Geometry: final body of the model. Coordinates: model frame, mm. A direction names the side the tool comes from. Round coordinates to 2 decimals unless told otherwise and drop trailing zeros. Loops run counter-clockwise (first coordinate to the right, second up) from the corner with the lowest first, then second, coordinate; pieces in that order, holes last. Notation, with made-up numbers: M -17,13.5 L 18,13.5 A18 cw 18,28.5 Z; hole C -34.75,-36.5 d10. An arc over 180 degrees is marked long. Return JSON: item names as keys, results as strings.
from build123d import *

# Parameters (mm, degrees)
F0_R     = 12.4944504689
F1_DEPTH = 25
F3_DEPTH = 20
F4_R     = 19.99999
F5_R     = 19.99999
F6_R     = 3.63588552
F7_DEPTH = 150.7420863042


# Not quite as in the source:
# - a fillet or chamfer is up to 0.001 mm smaller than in the source, because OpenCascade refuses the exact size


with BuildPart() as f1:
    # F0 (on Top) → F1 (new body)
    with BuildSketch(Plane.XY):
        with BuildLine():
            Line((-82.6911404729, -28.0499458313), (82.6911404729, -28.0499458313))
            ThreePointArc((82.6911404729, -28.0499458313), (110.7410863042, 0), (82.6911404729, 28.0499458313))
            Line((82.6911404729, 28.0499458313), (-82.6911404729, 28.0499458313))
            ThreePointArc((-82.6911404729, 28.0499458313), (-110.7410863042, 0), (-82.6911404729, -28.0499458313))
        make_face()
        with Locations((-82.6911404729, 0)):
            Circle(F0_R, mode=Mode.SUBTRACT)
        with Locations((82.6911404729, 0)):
            Circle(F0_R, mode=Mode.SUBTRACT)
    extrude(amount=F1_DEPTH)

    # F2 (on Front) → F3 (join, symmetric)
    with BuildSketch(Plane.XZ):
        Polygon((-40, 25), (40, 25), (40, 95), (20, 95), (20, 45), (-20, 45), (-20, 95), (-40, 95), align=None)
    extrude(amount=F3_DEPTH, both=True)

    # F4 (radius 20 in the source; OpenCascade refuses exactly that, so slightly less here)
    f4_edges = [f1.edges().sort_by_distance(p)[0] for p in [
        (-20, 0, 45),
        (20, 0, 45),
    ]]
    fillet(f4_edges, radius=F4_R)

    # F5 (radius 20 in the source; OpenCascade refuses exactly that, so slightly less here)
    f5_edges = [f1.edges().sort_by_distance(p)[0] for p in [
        (-30, -20, 95),
        (-30, 20, 95),
        (30, -20, 95),
        (30, 20, 95),
    ]]
    fillet(f5_edges, radius=F5_R)

    # F6 (on face) → F7 (cut, through all)
    with BuildSketch(Plane.YZ.offset(40)):
        with Locations((0, 75)):
            Circle(F6_R)
    extrude(amount=-F7_DEPTH, mode=Mode.SUBTRACT)


solid = f1.part
Q1. Section query C-C (z = 31.5). Output: boundary loops of the cut face in (x, y), plus the area to 3 significant figures.
Determined:
{"outline": "M -40,-20 L 40,-20 L 40,20 L -40,20 Z", "area": "3,200 mm^2"}
Q2. Pin query (flat end, axial travel): pin 1 (25 mm diameter, centred on x = 3, z = 50, fed in from +Y); pin 2 (20 mm diameter, centred on x = 82.69, y = 0, fed in from +Z) (1 decimal); pin 3 (3 mm diameter, centred on y = 10, z = 14, fed in from +X); pin 4 (5 mm diameter, centred on x = 7.5, z = 35, fed in from -Y). Return the tip coordinate at first contact, or that it passes through.
Determined:
{"pin 1": "stops at y = 20", "pin 2": "passes through", "pin 3": "stops at x = 109.42", "pin 4": "stops at y = -20"}
Q3. Section query D-D (x = 63.5). Output: boundary loops of the cut face in (y, z).
Determined:
{"outline": "M -28.05,0 L 28.05,0 L 28.05,25 L -28.05,25 Z"}
Q4. Section query A-A (x = -88). Output: boundary loops of the cut face in (y, z).
Determined:
{"outline": "M -27.54,0 L -11.31,0 L -11.31,25 L -27.54,25 Z; M 11.31,0 L 27.54,0 L 27.54,25 L 11.31,25 Z"}
Q5. Reachability of faces 1 (the flat face through (-40, 0, 60)), 2 (the flat face through (20, 0, 80)), 3 (the flat face through (40, 0, 60)), 4 (the flat face through (-0.6, 20, 44.8)) from +Z, -Z, +X, -X, +Y, -Y: full face, straight path, thin tool, end or side. Return the list, or none.
Determined:
{"face 1": "+Z, -X, +Y, -Y", "face 2": "+Z, +Y, -Y", "face 3": "+Z, +X, +Y, -Y", "face 4": "+Z, +X, -X, +Y"}
Q6. Material intervals for L1, parallel to X at y = 7.5, z = 79; L2, parallel to Y at x = 21.5, z = 75.5; L3, parallel to Y at x = 82, z = 16.5, sorted ascending.
Determined:
{"L1": "x = -40 to -20, 20 to 40", "L2": "y = -19.99 to -3.6, 3.6 to 19.99", "L3": "y = -28.05 to -12.48, 12.48 to 28.05"}
Q7. Pull-direction query (Z, two-part tool) for faces 5 (the cylindrical face through (-29.9, -0.5, 78.6)), 6 (the cylindrical face through (-13.986, -0.28, 50.703)), 7 (the flat face through (-2, 0, 0)); classes: pulls with the +Z half, pulls with the -Z half, needs draft (parallel to the pull), parting line crosses it, or undercut.
Determined:
{"face 5": "undercut", "face 6": "pulls with the +Z half", "face 7": "pulls with the -Z half"}
